from build123d import *

# Parameters (mm, degrees)
BOSS_EXTRUDE1_DEPTH = 12.7
BOSS_EXTRUDE2_START = -12.7
SKETCH3_W           = 28.575
SKETCH3_H           = 28.575
BOSS_EXTRUDE2_DEPTH = 28.575
SKETCH4_R           = 12.7
BOSS_EXTRUDE3_DEPTH = 28.575
BOSS_EXTRUDE4_DEPTH = 19.05
FILLET1_R           = 25.4


with BuildPart() as part:
    # Sketch1 → Revolve1 (revolve)
    with BuildSketch(Plane.XY, mode=Mode.PRIVATE) as revolve1_sk:
        with BuildLine():
            Line((0, 0), (165.1, 0))
            Line((165.1, 0), (165.1, 1143))
            add(Edge.make_bspline(
                [(165.1, 1143), (143.698147325, 1240.08378947), (52.321616657, 1282.7)],
                knots=[0, 0, 0, 1, 1, 1], degree=2))
            Line((52.321616657, 1282.7), (52.321616657, 1308.1))
            Line((52.321616657, 1308.1), (12.7, 1308.1))
            Line((12.7, 1308.1), (12.7, 1384.3))
            Line((12.7, 1384.3), (25.4, 1384.3))
            Line((25.4, 1384.3), (25.4, 1397))
            Line((25.4, 1397), (0, 1397))
            Line((0, 1397), (0, 0))
        make_face()
    revolve(revolve1_sk.sketch.rotate(Axis((0, 0, 0), (0, 1, 0)), 90), axis=Axis((0, 0, 0), (0, 1, 0)))

    # Sketch2 → Boss-Extrude1 (add)
    with BuildSketch(Plane(origin=(0, 1397, 0), x_dir=(1, 0, 0), z_dir=(0, 1, 0))):
        with BuildLine():
            ThreePointArc((-18.159539937, -17.759254187), (-12.7, -21.997045256), (-6.300195309, -24.60625))
            ThreePointArc((-6.300195309, -24.60625), (0, -31.75), (6.300195309, -24.60625))
            ThreePointArc((6.300195309, -24.60625), (12.7, -21.997045256), (18.159539937, -17.759254187))
            ThreePointArc((18.159539937, -17.759254187), (27.49630657, -15.875), (24.459735247, -6.846995813))
            ThreePointArc((24.459735247, -6.846995813), (25.4, 0), (24.459735247, 6.846995813))
            ThreePointArc((24.459735247, 6.846995813), (27.49630657, 15.875), (18.159539937, 17.759254187))
            ThreePointArc((18.159539937, 17.759254187), (12.7, 21.997045256), (6.300195309, 24.60625))
            ThreePointArc((6.300195309, 24.60625), (0, 31.75), (-6.300195309, 24.60625))
            ThreePointArc((-6.300195309, 24.60625), (-12.7, 21.997045256), (-18.159539937, 17.759254187))
            ThreePointArc((-18.159539937, 17.759254187), (-27.49630657, 15.875), (-24.459735247, 6.846995813))
            ThreePointArc((-24.459735247, 6.846995813), (-25.4, 0), (-24.459735247, -6.846995813))
            ThreePointArc((-24.459735247, -6.846995813), (-27.49630657, -15.875), (-18.159539937, -17.759254187))
        make_face()
    extrude(amount=-BOSS_EXTRUDE1_DEPTH)

    # Sketch3 → Boss-Extrude2 (add)
    with BuildSketch(Plane(origin=(0, 0, 0), x_dir=(0, 0, -1), z_dir=(1, 0, 0)).offset(BOSS_EXTRUDE2_START)):
        with Locations((0, 1325.5625)):
            Rectangle(SKETCH3_W, SKETCH3_H)
    extrude(amount=BOSS_EXTRUDE2_DEPTH)

    # Sketch4 → Boss-Extrude3 (add)
    with BuildSketch(Plane.XY):
        with Locations((0, 1358.9)):
            Circle(SKETCH4_R)
    extrude(amount=BOSS_EXTRUDE3_DEPTH)

    # Sketch5 → Boss-Extrude4 (add)
    with BuildSketch(Plane.XY.offset(28.575)):
        Polygon((14.664696837, 1358.9), (7.332348419, 1371.6), (-7.332348419, 1371.6), (-14.664696837, 1358.9), (-7.332348419, 1346.2), (7.332348419, 1346.2), align=None)
    extrude(amount=BOSS_EXTRUDE4_DEPTH)

    # Fillet1
    fillet1_edges = [part.edges().sort_by_distance(p)[0] for p in [
        (0, 0, 165.1),
    ]]
    fillet(fillet1_edges, radius=FILLET1_R)


solid = part.part
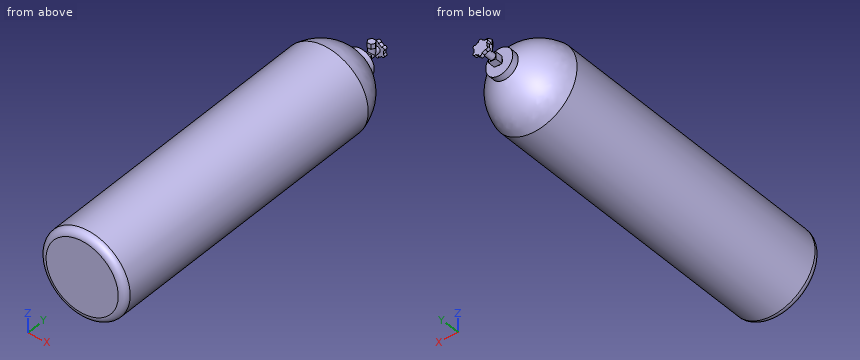
Design review of the part built by this model. Coordinates are the model's own, in mm. Give positions to 0.01 mm unless a question says otherwise; leave off trailing zeros. Write each loop counter-clockwise with the first axis right and the second up, starting at its lowest first coordinate (ties: lowest second). Pieces come first, ordered by that corner, then holes. Notation, with made-up numbers: M 62,59.25 L 81,59.25 A25 cw 81,76.25 Z; hole C -26,-11 d4. An arc over 180 degrees is marked long. Answer as a JSON object with one key per item and string values. Group by question number.
1) Clearance check with flat-ended pins moving along their axes: pin 1 Ø6 at (y, z) = (227.5, -85.5) entering from -X; pin 2 Ø3 at (x, y) = (5.5, 1349) entering from -Z; pin 3 Ø3 at (x, y) = (-12.5, 1355.5) entering from -Z. State where each tip first meets the part, or that it passes through.
2) For line 1 along Y through (x, z) = (-26.5, -28); line 2 along Z through (x, y) = (103, 613); line 3 along X through (y, z) = (562, 89), list the stretches that pass through material, from the lowest coordinate up.
3) We need section A-A (y = 670). Give the boundary of the cut face in (x, z), and give its area (3 significant figures).
Answer key:
{
 "1": {"pin 1": "stops at x = -143.01", "pin 2": "stops at z = -12.05", "pin 3": "stops at z = -6.35"},
 "2": {"line 1": "y = 0 to 1308.1", "line 2": "z = -129.03 to 129.03", "line 3": "x = -139.06 to 139.06"},
 "3": {"outline": "C 0,0 d330.2", "area": "85,600 mm²"}
}
